Autodesk Inventor part; units mm, degrees
ref_plane "YZ Plane" through (0, 0, 0) normal (1, 0, 0) x (0, 1, 0)
ref_plane "XZ Plane" through (0, 0, 0) normal (0, 1, 0) x (-1, 0, 0)
ref_plane "XY Plane" through (0, 0, 0) normal (0, 0, 1) x (1, 0, 0)
sketch "草圖1" plane through (0, 0, 0) normal (0, 0, 1) x (1, 0, 0)
  arc A0 (0.3, -2.4819) -> (-0.3, -2.4819) centre (0, 0) ccw
  arc A1 (0.3, -1.7241) -> (-0.3, -1.7241) centre (0, 0) ccw
  line L0 (0.3, -1.7241) -> (0.3, -2.4819)
  line L1 (-0.3, -2.4819) -> (-0.3, -1.7241)
  dimension "d0" = 5
  dimension "d1" = 3.5
  dimension "d2" = 0.3
  dimension "d3" = 0.6
extrude "擠出1" add sketch "草圖1" along normal blind 50
fillet "圓角1" radius 0.5 2 edges at (0, 2.5, 50) (0, 2.5, 0)
properties part number "5x65彈簧銷"
Design review of the part built by this model. Coordinates are the model's own, in mm. Round coordinates to 2 decimals unless told otherwise and drop trailing zeros. Order: outer loops, then holes, each group sorted by start corner. A loop starts at its lowest first (then second) coordinate and runs counter-clockwise, first axis right, second up. Notation, with made-up numbers: M 59,17.25 L 68,17.25 A24 cw 68,46.25 Z; hole C 81,-36.75 d4. An arc over 180 degrees is marked long. Put each result on its own line as item: value.
Q1. Consider section A-A (y = 0). State the section outline as (x, z) points.
Reported:
outline: M -2.5,0.5 A0.5 ccw -2,0 L -1.75,0 L -1.75,50 L -2,50 A0.5 ccw -2.5,49.5 Z; M 1.75,0 L 2,0 A0.5 ccw 2.5,0.5 L 2.5,49.5 A0.5 ccw 2,50 L 1.75,50 Z
Q2. Consider section B-B (z = 9). State the section outline as (x, y) points.
Reported:
outline: M -0.3,-2.48 L -0.3,-1.72 A1.75 cw long 0.3,-1.72 L 0.3,-2.48 A2.5 ccw long Z
Q3. Draft analysis for pull direction X (two halves, no side actions). For faces 1 (the face through (-0.106, 2.498, 24.657)), 2 (the face through (-0.07, 1.75, 24.65)), state which applies: released by +X, released by -X, zero draft, split by the parting line, or undercut.
Reported:
face 1: split by the parting line
face 2: undercut
Q4. To check wall thickness, follow line 1 (X direction, y = 0, z = 11); line 2 (Y direction, x = 1.2, z = 45); line 3 (Y direction, x = 0.15, z = 5.5). State the ranges of each line that lie inside material, in increasing order.
Reported:
line 1: -2.5 to -1.75, 1.75 to 2.5
line 2: -2.19 to -1.27, 1.27 to 2.19
line 3: 1.74 to 2.5
Q5. Insertion check: pin 1 Ø0.8 at (y, z) = (-2, 30.5) entering from -X; pin 2 Ø0.8 at (y, z) = (-2.5, 13) entering from +X; pin 3 Ø2 at (x, z) = (-1.5, 14) entering from -Y; pin 4 Ø1 at (x, y) = (1.5, 1.5) entering from -Z. Each pin has a flat end and moves straight along its axis. Give the tip position at first contact, or say it passes through.
Reported:
pin 1: x = -1.92
pin 2: x = 1.36
pin 3: y = -2.45
pin 4: z = 0
